Answer from the drawing. Dimensions are ordinates in mm from the lowest x, y and z of the part. A direction names the side the tool comes from. Round coordinates to 2 decimals unless told otherwise and drop trailing zeros. Write each loop counter-clockwise with the first axis right and the second up, starting at its lowest first coordinate (ties: lowest second). Pieces come first, ordered by that corner, then holes. Notation, with made-up numbers: (65.25, -30.5) - (77.25, -30.5) arc R23 cw to (77.25, -11.5) - close; hole circle Ø9 at (-21, -13.5). An arc over 180 degrees is marked (long way). Answer in a Markdown table with one row per item.
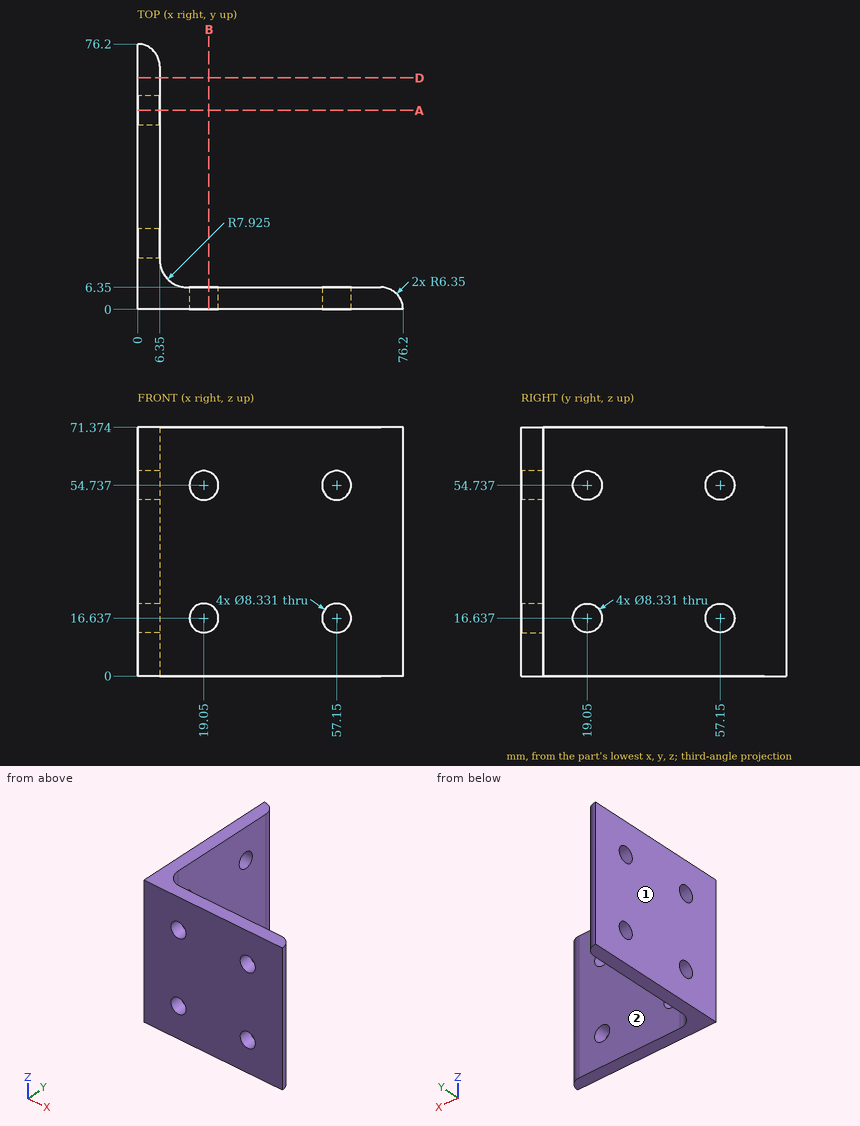
(1) For the marked faces 1 and 2, determine the directions among +Z, -Z, +X, -X, +Y, -Y from which every point of the face is accessible in a straight line to the end or side of a thin tool.
Checked values:
| item | result |
|---|---|
| face 1 | +Z, -Z, -X, +Y, -Y |
| face 2 | +Z, -Z, +X, +Y |
(2) Section A-A (y = 57.15) is taken. Give the vertices of the cut face in (x, z), and give its area (3 significant figures).
Checked values:
| item | result |
|---|---|
| outline | (0, 0) - (6.35, 0) - (6.35, 12.47) - (0, 12.47) - close; (0, 20.8) - (6.35, 20.8) - (6.35, 50.57) - (0, 50.57) - close; (0, 58.9) - (6.35, 58.9) - (6.35, 71.37) - (0, 71.37) - close |
| area | 347 mm2 |
(3) Section D-D (y = 66.5) is taken. Give the vertices of the cut face in (x, z), and give its area (3 significant figures).
Checked values:
| item | result |
|---|---|
| outline | (0, 0) - (6.35, 0) - (6.35, 71.37) - (0, 71.37) - close |
| area | 453 mm2 |
(4) Section B-B (x = 20.5) is taken. Give the vertices of the cut face in (y, z), and give its area (3 significant figures).
Checked values:
| item | result |
|---|---|
| outline | (0, 0) - (6.35, 0) - (6.35, 12.73) - (0, 12.73) - close; (0, 20.54) - (6.35, 20.54) - (6.35, 50.83) - (0, 50.83) - close; (0, 58.64) - (6.35, 58.64) - (6.35, 71.37) - (0, 71.37) - close |
| area | 354 mm2 |
(5) Flat-ended cylindrical pins translate along their axes: pin 1 (13.5 mm diameter, centred on x = 19.05, z = 54.737, fed in from +Y); pin 2 (5 mm diameter, centred on x = 33.5, z = 7.5, fed in from +Y); pin 3 (5 mm diameter, centred on x = 64.5, z = 13.5, fed in from +Y). Find the tip coordinate at first contact, or state that the pin passes through.
Checked values:
| item | result |
|---|---|
| pin 1 | stops at y = 6.6 |
| pin 2 | stops at y = 6.35 |
| pin 3 | stops at y = 6.35 |
(6) Find the intervals of material crossed by line 1 (Z direction, x = 57, y = 3); line 2 (Y direction, x = 49, z = 36.5), in increasing order.
Checked values:
| item | result |
|---|---|
| line 1 | z = 0 to 12.47, 20.8 to 50.57, 58.9 to 71.37 |
| line 2 | y = 0 to 6.35 |
